The listing builds one solid part. Answer for the finished solid, in the listing's coordinates (mm). A direction names the side the tool comes from. Round coordinates to 2 decimals unless told otherwise and drop trailing zeros. Loops run counter-clockwise (first coordinate to the right, second up) from the corner with the lowest first, then second, coordinate; pieces in that order, holes last. Notation, with made-up numbers: M -38,-32 L 16,-32 A20 ccw 16,-24 Z; hole C -32.75,-35.75 d11. An arc over 180 degrees is marked long. Put each result on its own line as item: value. Start each with the question number.
(1) Section C-C, the plane z = -29 is taken. Determine the outline of the cut face in (x, y), then the cut area to 3 significant figures.
(2) Determine the mould class of faces 1 (the face through (3, 20, -35)), 2 (the face through (17.2, 40, -4.6)), 3 (the face through (3, 29, -11)) for opening direction Z: released by +Z, released by -Z, zero draft, split by the parting line, or undercut.
(3) Section B-B, the plane x = 49.2 is taken. Determine the outline of the cut face in (y, z), then the cut area to 3 significant figures.
(4) Flat-ended cylindrical pins translate along their axes: P1, Ø1.5, axis at y = 6.5, z = -13.5, coming from the +X side; P2, Ø3, axis at x = 38, y = 11.5, coming from the -Z side. Find the tip coordinate at first contact, or state that the pin passes through.
(5) Straight lines are drawn through the part: line 1 (Y direction, x = 2.7, z = -11); line 2 (Y direction, x = 40, z = -3); line 3 (Y direction, x = 30.8, z = -2.1). For each, find the intervals that lie inside material, in ascending order.
(6) Which of the six approach directions +Z, -Z, +X, -X, +Y, -Y give full straight-line access (tool end or side, diameter ignored) to faces 4 (the face through (7, 5, -7)), 5 (the face through (37.136, 10.813, -2.535))?
(7) Section A-A, the plane y = 20 is taken. Determine the outline of the cut face in (x, z).
(8) Section D-D, the plane z = -11 is taken. Determine the outline of the cut face in (x, y).
```python
from build123d import *

# Parameters (mm, degrees)
BOSS_EXTRUDE3_DEPTH = 40
CUT_EXTRUDE1_DEPTH  = 35
BOSS_EXTRUDE4_DEPTH = 5
SKETCH7_R           = 2
SKETCH7_R_2         = 3.1
SKETCH7_R_3         = 2.1
CUT_EXTRUDE7_DEPTH  = 5
SKETCH15_R          = 2
CUT_EXTRUDE8_DEPTH  = 73.972597597


with BuildPart() as part:
    # Sketch1 → Boss-Extrude3 (new body)
    with BuildSketch(Plane(origin=(0, 0, 0), x_dir=(1, 0, 0), z_dir=(0, 1, 0))):
        Polygon((0, 0), (55, 0), (55, 5), (13.75, 5), (5, 13.75), (5, 35), (0, 35), align=None)
    extrude(amount=BOSS_EXTRUDE3_DEPTH)

    # Sketch5 → Cut-Extrude1 (cut)
    with BuildSketch(Plane.XZ):
        Polygon((5, -13.75), (5, -5), (13.75, -5), align=None)
    extrude(amount=-CUT_EXTRUDE1_DEPTH, mode=Mode.SUBTRACT)

    # Sketch6 → Boss-Extrude4 (add)
    with BuildSketch(Plane.XZ):
        Polygon((13.75, -5), (5, -13.75), (5, -5), align=None)
    extrude(amount=-BOSS_EXTRUDE4_DEPTH)

    # Sketch7 → Cut-Extrude7 (cut)
    with BuildSketch(Plane(origin=(0, 0, -5), x_dir=(-1, 0, 0), z_dir=(0, 0, -1))):
        with Locations((-49.2, 32)):
            Circle(SKETCH7_R)
        with Locations((-40, 12)):
            Circle(SKETCH7_R_2)
        with Locations((-40, 23)):
            Circle(SKETCH7_R_3)
        with Locations((-30.8, 32)):
            Circle(SKETCH7_R)
    extrude(amount=-CUT_EXTRUDE7_DEPTH, mode=Mode.SUBTRACT)

    # Sketch15 → Cut-Extrude8 (cut, through all)
    with BuildSketch(Plane(origin=(5, 0, 0), x_dir=(0, 0, -1), z_dir=(1, 0, 0))):
        with Locations((11, 31)):
            Circle(SKETCH15_R)
        with Locations((11, 9)):
            Circle(SKETCH15_R)
        with Locations((29, 20)):
            Circle(SKETCH15_R)
    extrude(amount=-CUT_EXTRUDE8_DEPTH, mode=Mode.SUBTRACT)


solid = part.part
```
Recorded:
1. outline: M 0,0 L 5,0 L 5,18 L 0,18 Z; M 0,22 L 5,22 L 5,40 L 0,40 Z
1. area: 180 mm²
2. face 1: released by -Z
2. face 2: zero draft
2. face 3: undercut
3. outline: M 0,-5 L 30,-5 L 30,0 L 0,0 Z; M 34,-5 L 40,-5 L 40,0 L 34,0 Z
3. area: 180 mm²
4. P1: stops at x = 5
4. P2: stops at z = -5
5. line 1: y = 0 to 7, 11 to 29, 33 to 40
5. line 2: y = 0 to 8.9, 15.1 to 20.9, 25.1 to 40
5. line 3: y = 0 to 30, 34 to 40
6. face 4: -Z, +X
6. face 5: +Z, -Z
7. outline: M 0,-35 L 5,-35 L 5,-31 L 0,-31 Z; M 0,-27 L 5,-27 L 5,-5 L 55,-5 L 55,0 L 0,0 Z
8. outline: M 0,0 L 7.75,0 L 7.75,5 L 5,5 L 5,7 L 0,7 Z; M 0,11 L 5,11 L 5,29 L 0,29 Z; M 0,33 L 5,33 L 5,35 L 7.75,35 L 7.75,40 L 0,40 Z
